Study the drawing (mm; zero at the part's minimum x, y, z) and answer. A direction names the side the tool comes from. Give positions to 0.01 mm unless a question says otherwise; leave off trailing zeros. Write each loop counter-clockwise with the first axis right and the second up, starting at its lowest first coordinate (ties: lowest second). Pieces come first, ordered by that corner, then holes. Notation, with made-up numbers: M 84,10 L 89,10 A14 ccw 89,16 Z; hole C 71,64.5 d1. An arc over 180 degrees is marked long. Use a Markdown table: item, result. Add a question column.
Item 1: A cutting plane is placed at D-D on y = 6.5. Determine the outline of the cut face in (x, z), then the cut area to 3 significant figures.
Item 2: A cutting plane is placed at A-A on z = 50. Determine the outline of the cut face in (x, y).
Item 3: A cutting plane is placed at C-C on x = 65. Determine the outline of the cut face in (y, z), then the cut area to 3 significant figures.
Item 4: A cutting plane is placed at B-B on x = 15. Determine the outline of the cut face in (y, z).
Item 5: Given P1, Ø2, axis at x = 27, y = 29.5, coming from the -Z side; P2, Ø4, axis at x = 22.5, y = 25, coming from the -Z side; P3, Ø10, axis at y = 69.5, z = 32, coming from the -X side; P4, Ø5.5, axis at x = 15, z = 73.25, coming from the -Y side, each flat-ended and moving along its own axis, determine where each tip first touches the part or whether it passes through.
Item 6: The mould has two halves that part along X. Classify the marked faces 3, 4, 5 and 6: pulls with the +X half, pulls with the -X half, needs draft (parallel to the pull), parting line crosses it, or undercut.
Item 7: For the marked faces 1 and 2, determine the directions among +Z, -Z, +X, -X, +Y, -Y from which every point of the face is accessible in a straight line to the end or side of a thin tool.
Item 8: Consider probe 1 along Z at (x, y) = (115, 5.5); probe 2 along Z at (x, y) = (65, 49.5); probe 3 along X at (y, z) = (61.5, 49). Determine where each line is inside the solid, lowest interval first. Write a range as [from, to].
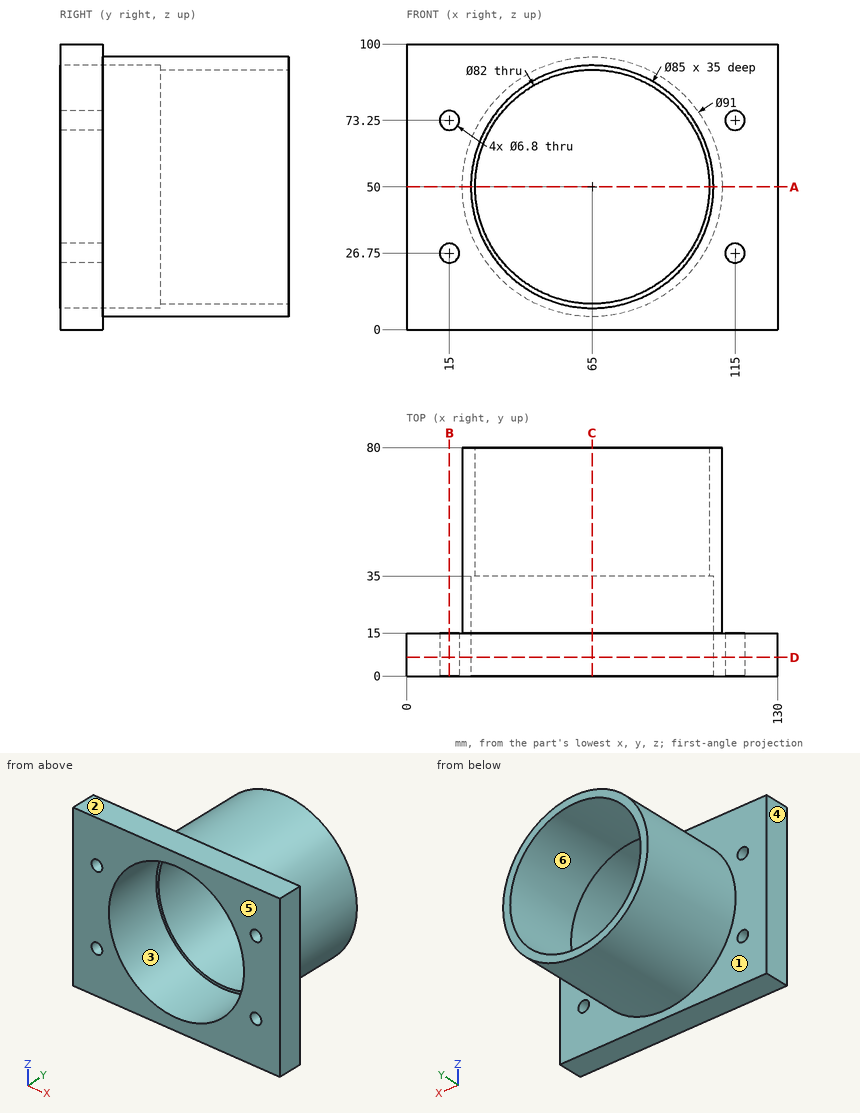
Filled in:
| question | item | result |
|---|---|---|
| 1 | outline | M 0,0 L 130,0 L 130,100 L 0,100 Z; hole C 15,26.75 d6.8; hole C 15,73.25 d6.8; hole C 65,50 d85; hole C 115,26.75 d6.8; hole C 115,73.25 d6.8 |
| 1 | area | 7,180 mm² |
| 2 | outline | M 0,0 L 22.5,0 L 22.5,35 L 24,35 L 24,80 L 19.5,80 L 19.5,15 L 0,15 Z; M 106,35 L 107.5,35 L 107.5,0 L 130,0 L 130,15 L 110.5,15 L 110.5,80 L 106,80 Z |
| 3 | outline | M 0,0 L 15,0 L 15,4.5 L 80,4.5 L 80,9 L 35,9 L 35,7.5 L 0,7.5 Z; M 0,92.5 L 35,92.5 L 35,91 L 80,91 L 80,95.5 L 15,95.5 L 15,100 L 0,100 Z |
| 3 | area | 750 mm² |
| 4 | outline | M 0,0 L 15,0 L 15,23.35 L 0,23.35 Z; M 0,30.15 L 15,30.15 L 15,69.85 L 0,69.85 Z; M 0,76.65 L 15,76.65 L 15,100 L 0,100 Z |
| 5 | P1 | z = 23.52 |
| 5 | P2 | z = 29.26 |
| 5 | P3 | x = 21.4 |
| 5 | P4 | through |
| 6 | face 3 | undercut |
| 6 | face 4 | pulls with the -X half |
| 6 | face 5 | needs draft |
| 6 | face 6 | undercut |
| 7 | face 1 | +Y |
| 7 | face 2 | +Z, +X, -X, +Y, -Y |
| 8 | probe 1 | [0, 23.35], [30.15, 69.85], [76.65, 100] |
| 8 | probe 2 | [4.5, 9], [91, 95.5] |
| 8 | probe 3 | [19.51, 24.01], [105.99, 110.49] |
